Read the model definition and answer for the solid it produces. Units are mm, in the model's axes. Face numbers are marked on the shaded views. A direction names the side the tool comes from. Coordinates: 2 decimals unless noted, no trailing zeros. Write each loop counter-clockwise with the first axis right and the second up, starting at its lowest first coordinate (ties: lowest second). Pieces come first, ordered by that corner, then holes. Notation, with made-up numbers: (88, 65) -> (130, 65) arc R13 cw to (130, 90) -> close; hole circle Ø9 at (55, 67). An arc over 180 degrees is marked (long way). Return JSON: item names as keys, results as strings.
from build123d import *

# Parameters (mm, degrees)
SKETCH1_W                           = 54.5
SKETCH1_H                           = 111
BOSS_EXTRUDE1_DEPTH                 = 4.5
SKETCH2_W                           = 13.5
SKETCH2_H                           = 111
BOSS_EXTRUDE2_DEPTH                 = 12.5
M4X0_7_TAPPED_HOLE1_D               = 3.3
SKETCH6_W                           = 4
SKETCH6_H                           = 12.5
BOSS_EXTRUDE3_DEPTH                 = 37
SKETCH7_W                           = 54.5
SKETCH7_H                           = 3
BOSS_EXTRUDE5_DEPTH                 = 45
SKETCH8_R                           = 7
CUT_EXTRUDE1_DEPTH                  = 3
M2_CLEARANCE_HOLE1_D                = 2.4
F_8_0_199_DIAMETER_HOLE1_D          = 5.0546
SKETCH12_R                          = 5.5
CUT_EXTRUDE3_DEPTH                  = 3
SKETCH13_W                          = 27.5
SKETCH13_H                          = 9.513667368
CUT_EXTRUDE4_DEPTH                  = 5
SKETCH14_W                          = 54.5
SKETCH14_H                          = 6
BOSS_EXTRUDE6_DEPTH                 = 30
RIB6_REACH                          = 124.903
SKETCH20_WALL_W                     = 286.858082508
SKETCH20_WALL_H                     = 10
TAP_START                           = 50.370687416
TAP_DRILL_FOR_M4X0_7_TAP1_OUTLINE_R = 1.65
TAP_DRILL_FOR_M4X0_7_TAP1_DEPTH     = 6
TAP_START_2                         = -40.649543841
TAP_DRILL_FOR_M4X0_7_TAP1_2_DEPTH   = 10


with BuildPart() as part:
    # Sketch1 → Boss-Extrude1 (new body)
    with BuildSketch(Plane(origin=(0, 0, 0), x_dir=(1, 0, 0), z_dir=(0, 1, 0))):
        with Locations((-13.399543841, 44.129312584)):
            Rectangle(SKETCH1_W, SKETCH1_H)
    extrude(amount=BOSS_EXTRUDE1_DEPTH)

    # Sketch2 → Boss-Extrude2 (add)
    with BuildSketch(Plane(origin=(0, 4.5, 0), x_dir=(1, 0, 0), z_dir=(0, 1, 0))):
        with Locations((7.100456159, 44.129312584)):
            Rectangle(SKETCH2_W, SKETCH2_H)
        with Locations((-33.899543841, 44.129312584)):
            Rectangle(SKETCH2_W, SKETCH2_H)
    extrude(amount=BOSS_EXTRUDE2_DEPTH)

    # M4x0.7 Tapped Hole1 (through all)
    with Locations(Plane(origin=(-31.949543841, 17, -9.129312584), x_dir=(0, 0, 1), z_dir=(0, 1, 0))):
        with Locations((0, 0), (-25, 0), (-50, 0), (-75, 0), (0, 37.1), (-25, 37.1), (-50, 37.1), (-75, 37.1)):
            Hole(M4X0_7_TAPPED_HOLE1_D / 2)

    # Sketch6 → Boss-Extrude3 (add)
    with BuildSketch(Plane(origin=(-27.149543841, 0, 0), x_dir=(0, 0, -1), z_dir=(1, 0, 0))):
        with Locations((-9.370687416, 10.75)):
            Rectangle(SKETCH6_W, SKETCH6_H)
    extrude(amount=BOSS_EXTRUDE3_DEPTH)

    # Sketch7 → Boss-Extrude5 (add)
    with BuildSketch(Plane.XY.offset(11.370687416)):
        with Locations((-13.399543841, 15.5)):
            Rectangle(SKETCH7_W, SKETCH7_H)
    extrude(amount=BOSS_EXTRUDE5_DEPTH)

    # Sketch8 → Cut-Extrude1 (cut)
    with BuildSketch(Plane(origin=(0, 17, 0), x_dir=(1, 0, 0), z_dir=(0, 1, 0))):
        with Locations(Location((-13.399543841, -30.870687416, 0), (0, 0, 270))):
            Circle(SKETCH8_R)
    extrude(amount=-CUT_EXTRUDE1_DEPTH, mode=Mode.SUBTRACT)

    # M2 Clearance Hole1 (through all)
    with Locations(Plane(origin=(-20.200285158, 17, 29.83376219), x_dir=(0, 0, 1), z_dir=(0, 1, 0))):
        with Locations((0, 0), (-6.963074774, 6.800741317), (9.036925226, 6.800741317), (-0.001679632, 13.599250141)):
            Hole(M2_CLEARANCE_HOLE1_D / 2)

    # #8 (0.199) Diameter Hole1 (through all)
    with Locations(Plane(origin=(-13.399543841, 4.5, 2.370687416), x_dir=(0, 0, 1), z_dir=(0, 1, 0))):
        with Locations((0, 0), (-10, 0), (-35, 0), (-85, 0), (-95, 0)):
            Hole(F_8_0_199_DIAMETER_HOLE1_D / 2)

    # Sketch12 → Cut-Extrude3 (cut)
    with BuildSketch(Plane(origin=(0, 0, 0), x_dir=(-1, 0, 0), z_dir=(0, -1, 0))):
        with Locations(Location((13.399543841, 92.629312584, 0), (0, 0, 90))):
            Circle(SKETCH12_R)
    extrude(amount=-CUT_EXTRUDE3_DEPTH, mode=Mode.SUBTRACT)

    # Sketch13 → Cut-Extrude4 (cut)
    with BuildSketch(Plane.XY.offset(11.370687416)):
        with Locations((-13.399543841, 9.243166316)):
            Rectangle(SKETCH13_W, SKETCH13_H)
    extrude(amount=-CUT_EXTRUDE4_DEPTH, mode=Mode.SUBTRACT)

    # Sketch14 → Boss-Extrude6 (add)
    with BuildSketch(Plane(origin=(0, 17, 0), x_dir=(1, 0, 0), z_dir=(0, 1, 0))):
        with Locations((-13.399543841, -53.370687416)):
            Rectangle(SKETCH14_W, SKETCH14_H)
    extrude(amount=BOSS_EXTRUDE6_DEPTH)

    # Sketch20 wall → Rib6 (add, up to next)
    with BuildSketch(Plane(origin=(13.850456159, 32, 37.870687416), x_dir=(0, -0.768221279597, -0.640184399664), z_dir=(0, 0.640184399664, -0.768221279597)), mode=Mode.PRIVATE) as rib6_sk1:
        with Locations((0, 5)):
            Rectangle(SKETCH20_WALL_W, SKETCH20_WALL_H)
    rib6_tool1 = extrude(rib6_sk1.sketch, amount=-RIB6_REACH, mode=Mode.PRIVATE) - part.part
    add(rib6_tool1.solids().sort_by_distance((13.850456159, 32, 37.870687416))[0])

    # Tap Drill for M4x0.7 Tap1: read off the stored shape, not the designer's step
    # Tap Drill for M4x0.7 Tap1 outline → Tap Drill for M4x0.7 Tap1 (cut)
    with BuildSketch(Plane.XY.offset(TAP_START)):
        with Locations((-13.399543841, 30.5)):
            Circle(TAP_DRILL_FOR_M4X0_7_TAP1_OUTLINE_R)
        with Locations((-13.399543841, 38.75)):
            Circle(TAP_DRILL_FOR_M4X0_7_TAP1_OUTLINE_R)
        with Locations((-13.399543841, 22.25)):
            Circle(TAP_DRILL_FOR_M4X0_7_TAP1_OUTLINE_R)
    extrude(amount=TAP_DRILL_FOR_M4X0_7_TAP1_DEPTH, mode=Mode.SUBTRACT)

    # Tap Drill for M4x0.7 Tap1 2 outline → Tap Drill for M4x0.7 Tap1 2 (add)
    with BuildSketch(Plane.YZ.offset(TAP_START_2)):
        Polygon((17, 50.370687416), (17, 25.370687416), (47, 50.370687416), align=None)
    extrude(amount=TAP_DRILL_FOR_M4X0_7_TAP1_2_DEPTH)


solid = part.part
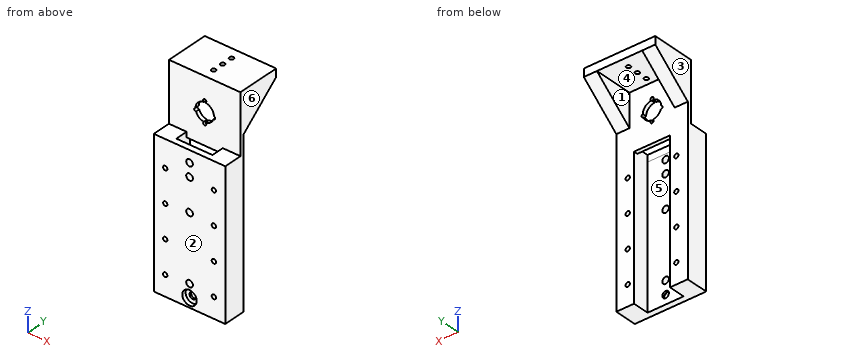
1. A tool of negligible diameter and unlimited length cuts with its end or side. For the marked faces 4, 5 and 6, from which of +Z, -Z, +X, -X, +Y, -Y can it reach the whole face along a straight path? Write none if from no direction.
Taken from the geometry:
{"face 4": "-Z, +Y", "face 5": "+Z, -Z, +Y", "face 6": "+Z, -Z, +X, +Y, -Y"}
2. Consider L1, parallel to X at y = 28.5, z = 35; L2, parallel to Y at x = 9, z = -26.5; L3, parallel to X at y = 8.5, z = 11. Determine where each line is inside the solid, lowest interval first.
Taken from the geometry:
{"L1": "x = -40.65 to -30.65, 3.85 to 13.85", "L2": "y = 0 to 17", "L3": "x = -40.65 to -27.15, 0.35 to 13.85"}
3. The part is cut by section B-B (y = 38.75). Determine the outline of the cut face in (x, z).
Taken from the geometry:
{"outline": "(-40.65, 43.5) -> (-30.65, 43.5) -> (-30.65, 50.37) -> (-15.05, 50.37) -> (-15.05, 56.37) -> (-40.65, 56.37) -> close; (-11.75, 50.37) -> (3.85, 50.37) -> (3.85, 43.5) -> (13.85, 43.5) -> (13.85, 56.37) -> (-11.75, 56.37) -> close"}
4. Flat-ended cylindrical pins translate along their axes: pin 1 Ø4.5 at (x, z) = (5.15, -84.13) entering from +Y; pin 2 Ø5.5 at (x, z) = (-31.95, -84.13) entering from -Y; pin 3 Ø12 at (x, y) = (5.5, 32) entering from -Z; pin 4 Ø12 at (x, y) = (-4, 25.5) entering from -Z. Find the tip coordinate at first contact, or state that the pin passes through.
Taken from the geometry:
{"pin 1": "stops at y = 17", "pin 2": "stops at y = 0", "pin 3": "stops at z = 32.87", "pin 4": "stops at z = 50.37"}
5. The part is cut by section D-D (y = 11.5). Count the separate pieces of the cut face and the enclosed holes in it, then the cut area to 3 significant figures.
Taken from the geometry:
{"separate pieces": "2", "enclosed holes": "8", "area": "2,930 mm2"}
6. The part is cut by section C-C (z = -15.5). Determine the outline of the cut face in (x, y), then the cut area to 3 significant figures.
Taken from the geometry:
{"outline": "(-40.65, 0) -> (13.85, 0) -> (13.85, 17) -> (0.35, 17) -> (0.35, 4.5) -> (-27.15, 4.5) -> (-27.15, 17) -> (-40.65, 17) -> close", "area": "583 mm2"}
7. For a pull along X with two mould halves and no side action, classify the marked faces 1, 2 and 3 as +X half, -X half, draft (parallel to the pull), parting line (faces both ways), or undercut.
Taken from the geometry:
{"face 1": "undercut", "face 2": "draft", "face 3": "-X half"}
